Could you check a few things on this model? Use its own coordinates, in mm. Round coordinates to 2 decimals unless told otherwise and drop trailing zeros. Order: outer loops, then holes, each group sorted by start corner. A loop starts at its lowest first (then second) coordinate and runs counter-clockwise, first axis right, second up. Notation, with made-up numbers: (24, 50.25) -> (50, 50.25) arc R27 cw to (50, 80.25) -> close; hole circle Ø3 at (36.25, -22.75). An arc over 180 degrees is marked (long way). One line per question, with ' | ' between items.
```python
from build123d import *

# Parameters (mm, degrees)
SKETCH1_W           = 200
SKETCH1_H           = 200
BOSS_EXTRUDE1_DEPTH = 8
SKETCH2_R           = 6
CUT_EXTRUDE1_DEPTH  = 142.647449677
SKETCH3_R           = 7.5
CUT_EXTRUDE2_DEPTH  = 142.647449677


with BuildPart() as part:
    # Sketch1 → Boss-Extrude1 (new body)
    with BuildSketch(Plane(origin=(0, 0, 0), x_dir=(0, 1, 0), z_dir=(0, 0, 1))):
        Rectangle(SKETCH1_W, SKETCH1_H)
    extrude(amount=BOSS_EXTRUDE1_DEPTH)

    # Sketch2 → Cut-Extrude1 (cut, through all)
    with BuildSketch(Plane(origin=(0, 0, 0), x_dir=(0, 1, 0), z_dir=(0, 0, 1))):
        with Locations(Location((-55, 55, 0), (0, 0, 270))):
            Circle(SKETCH2_R)
        with Locations(Location((55, 55, 0), (0, 0, 270))):
            Circle(SKETCH2_R)
        with Locations(Location((-55, -55, 0), (0, 0, 270))):
            Circle(SKETCH2_R)
        with Locations(Location((55, -55, 0), (0, 0, 270))):
            Circle(SKETCH2_R)
    extrude(amount=CUT_EXTRUDE1_DEPTH, mode=Mode.SUBTRACT)

    # Sketch3 → Cut-Extrude2 (cut, through all)
    with BuildSketch(Plane(origin=(0, 0, 0), x_dir=(0, 1, 0), z_dir=(0, 0, 1))):
        with Locations(Location((0, 0, 0), (0, 0, 270))):
            Circle(SKETCH3_R)
    extrude(amount=CUT_EXTRUDE2_DEPTH, mode=Mode.SUBTRACT)


solid = part.part
```
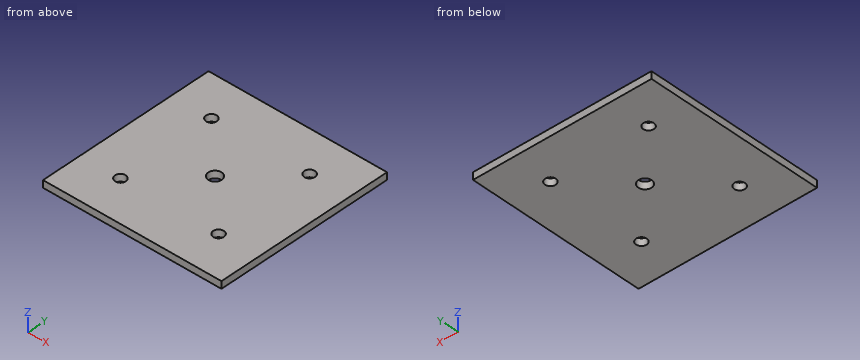
1. I'm going to push a flat-ended pin straight in: pin 1 (7 mm diameter, centred on x = -55, y = -55, fed in from +Z). Where does the tip first touch, or does it pass through?
From the geometry:
pin 1: passes through
2. I need wall thicknesses on probe 1 along X at (y, z) = (55, 6.25); probe 2 along Y at (x, z) = (0, 5.5). Which ranges of each line are inside material? Lowest first, please.
From the geometry:
probe 1: x = -100 to -61, -49 to 49, 61 to 100 | probe 2: y = -100 to -7.5, 7.5 to 100
3. I want a section at A-A on x = -55. List the corners of the cut face in (y, z) for me, and give its area (3 significant figures).
From the geometry:
outline: (-100, 0) -> (-61, 0) -> (-61, 8) -> (-100, 8) -> close; (-49, 0) -> (49, 0) -> (49, 8) -> (-49, 8) -> close; (61, 0) -> (100, 0) -> (100, 8) -> (61, 8) -> close | area: 1,410 mm²
4. I want a section at D-D on z = 4.5. List the corners of the cut face in (x, y) for me, and give its area (3 significant figures).
From the geometry:
outline: (-100, -100) -> (100, -100) -> (100, 100) -> (-100, 100) -> close; hole circle Ø12 at (-55, -55); hole circle Ø12 at (-55, 55); hole circle Ø15 at (0, 0); hole circle Ø12 at (55, -55); hole circle Ø12 at (55, 55) | area: 39,400 mm²
5. I want a section at B-B on x = 0. List the corners of the cut face in (y, z) for me.
From the geometry:
outline: (-100, 0) -> (-7.5, 0) -> (-7.5, 8) -> (-100, 8) -> close; (7.5, 0) -> (100, 0) -> (100, 8) -> (7.5, 8) -> close
